Work out the finished part from the listing and answer in its coordinate system (mm). Face numbers are marked on the shaded views. A direction names the side the tool comes from. Give positions to 0.01 mm unless a question says otherwise; leave off trailing zeros. Loops run counter-clockwise (first coordinate to the right, second up) from the corner with the lowest first, then second, coordinate; pieces in that order, holes last. Notation, with made-up numbers: (33, 21) -> (69, 21) arc R16 ccw to (69, 26) -> close; hole circle Ø8 at (45, -27). An arc over 180 degrees is marked (long way). Answer as CSV lines item,"result". Start each with the question number.
1. Find section A-A, the plane z = 6. Give the vertices of the cut face in (x, y), and give its area (3 significant figures).
2. Determine the mould class of the marked faces 1, 2 and 3 for opening direction Y: +Y half, -Y half, draft (parallel to the pull), parting line (faces both ways), or undercut.
3. Find the intervals of material crossed by line 1 along X through (y, z) = (12.5, 3.75); line 2 along Y through (x, z) = (38.5, 8); line 3 along X through (y, z) = (26, 4), in increasing order.
4. Find section B-B, the plane y = 50.5. Give the vertices of the cut face in (x, z).
5. Flat-ended cylindrical pins translate along their axes: pin 1 Ø6 at (x, y) = (28.5, 39.5) entering from +Z; pin 2 Ø11.5 at (x, y) = (0.08, 18.28) entering from -Z; pin 3 Ø2 at (x, y) = (17.5, -8.5) entering from -Z. Find the tip coordinate at first contact, or state that the pin passes through.
6. Find section C-C, the plane x = -40.5. Give the vertices of the cut face in (y, z).
7. A tool of negligible diameter and unlimited length cuts with its end or side. For the marked faces 4 and 5, from which of +Z, -Z, +X, -X, +Y, -Y can it reach the whole face along a straight path? Write none if from no direction.
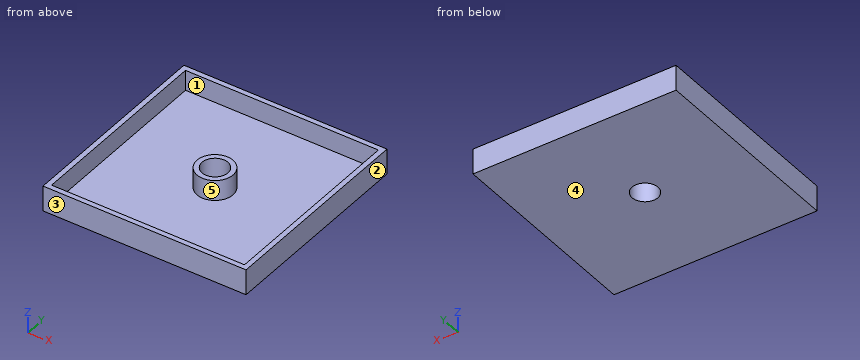
from build123d import *

# Parameters (mm, degrees)
F0_W     = 101.6
F0_H     = 101.6
F0_R     = 6.477
F1_DEPTH = 12.7
F2_T     = -2.54


with BuildPart() as f1:
    # F0 (on Top) → F1 (new body)
    with BuildSketch(Plane.XY):
        with Locations((0.083563, 18.284834)):
            Rectangle(F0_W, F0_H)
        with Locations((0.083563, 18.284834)):
            Circle(F0_R, mode=Mode.SUBTRACT)
    extrude(amount=F1_DEPTH)

    # F2
    f2_openings = [f1.faces().sort_by_distance(p)[0] for p in [
        (49.446723, 18.284834, 12.7),
    ]]
    offset(amount=F2_T, openings=f2_openings)


solid = f1.part
Resolved:
1,outline,"(-50.72, -32.52) -> (50.88, -32.52) -> (50.88, 69.08) -> (-50.72, 69.08) -> close; circle Ø18.03 at (0.08, 18.28); hole (-48.18, -29.98) -> (48.34, -29.98) -> (48.34, 66.54) -> (-48.18, 66.54) -> close; hole circle Ø12.95 at (0.08, 18.28)"
1,area,"1,130 mm^2"
2,face 1,"undercut"
2,face 2,"draft"
2,face 3,"-Y half"
3,line 1,"x = -50.72 to -48.18, -6.83 to -2.83, 3 to 7, 48.34 to 50.88"
3,line 2,"y = -32.52 to -29.98, 66.54 to 69.08"
3,line 3,"x = -50.72 to -48.18, -4.58 to 4.75, 48.34 to 50.88"
4,outline,"(-50.72, 0) -> (50.88, 0) -> (50.88, 12.7) -> (48.34, 12.7) -> (48.34, 2.54) -> (-48.18, 2.54) -> (-48.18, 12.7) -> (-50.72, 12.7) -> close"
5,pin 1,"stops at z = 2.54"
5,pin 2,"passes through"
5,pin 3,"stops at z = 0"
6,outline,"(-32.52, 0) -> (69.08, 0) -> (69.08, 12.7) -> (66.54, 12.7) -> (66.54, 2.54) -> (-29.98, 2.54) -> (-29.98, 12.7) -> (-32.52, 12.7) -> close"
7,face 4,"-Z, +X, -X, +Y, -Y"
7,face 5,"+Z"
